Here's how the part is built. I have some questions about the finished solid (model axes, mm). A direction names the side the tool comes from. Coordinates: 2 decimals unless noted, no trailing zeros. Write each loop counter-clockwise with the first axis right and the second up, starting at its lowest first coordinate (ties: lowest second). Pieces come first, ordered by that corner, then holes. Notation, with made-up numbers: (83, 6.5) -> (107, 6.5) arc R16 ccw to (107, 10.5) -> close; hole circle Ø5 at (-24.5, -32.5). An arc over 180 degrees is marked (long way). Use a Markdown table: item, result. Add a question column.
Item 1: Imagine slicing it at C-C, the plane z = 0.3. Write out the boundary of the cut face in (x, y).
Item 2: Imagine slicing it at D-D, the plane x = 8. Write out the boundary of the cut face in (y, z).
Item 3: If we mould it in two halves opening along Y, with no side actions, what happens to faces 1 (the cylindrical face through (39.7, -10.9, 0.9)), 2 (the flat face through (36.79, 10.57, 0.89)), 3 (the flat face through (-15.78, 3, 1))? For each: pulls with the +Y half, pulls with the -Y half, needs draft (parallel to the pull), parting line crosses it, or undercut.
Item 4: Imagine slicing it at A-A, the plane x = 40. Write out the boundary of the cut face in (y, z).
Item 5: If I drill on line 1 along X through (y, z) = (-6, 0.1); line 2 along Y through (x, z) = (-9, 1.4); line 3 along Y through (x, z) = (45, 1.15) (3 decimals), over which ranges is the centre line in solid material (lowest first)? Write a range as from..to.
Item 6: Imagine slicing it at B-B, the plane y = -4. Write out the boundary of the cut face in (x, z).
Item 7: Will these pins go through, and if not, where does the flat tip stop? pin 1 Ø1 at (x, z) = (17, 0.5) entering from -Y; pin 2 Ø1 at (y, z) = (-1.5, 0) entering from +X; pin 3 Ø0.5 at (x, z) = (2.5, 1) entering from -Y.
Item 8: On a 3-axis mill with a long thin cutter (end or side, diameter ignored), from which of +Z, -Z, +X, -X, +Y, -Y can I reach the whole of each face in a straight line? I mean faces 4 (the flat face through (4, 15.405, 1)), 5 (the flat face through (-3, -9.595, 1)). Say none if no direction works.
```python
from build123d import *

# Parameters (mm, degrees)
RESSALTO_EXTRUS_O3_DEPTH = 1.8
ESBO_O7_R                = 5
CORTE_EXTRUS_O5_DEPTH    = 3


with BuildPart() as part:
    # Esboço1 → Ressalto-extrusão3 (new body)
    with BuildSketch(Plane.XY):
        with BuildLine():
            Line((-15.780332987, 15.405349819), (25.337197849, 15.405349819))
            Line((25.337197849, 15.405349819), (48.575213244, 5.595781738))
            ThreePointArc((48.575213244, 5.595781738), (51.52798537, -14.949789194), (30.790948881, -15.852377581))
            Line((30.790948881, -15.852377581), (9.828194525, -9.594650181))
            Line((9.828194525, -9.594650181), (-15.780332987, -9.594650181))
            Line((-15.780332987, -9.594650181), (-15.780332987, 15.405349819))
        make_face()
    extrude(amount=RESSALTO_EXTRUS_O3_DEPTH)

    # Esboço7 → Corte-extrusão5 (cut)
    with BuildSketch(Plane.XY.offset(1.8)):
        with Locations((40.750876667, -6.013686688)):
            Circle(ESBO_O7_R)
    extrude(amount=-CORTE_EXTRUS_O5_DEPTH, mode=Mode.SUBTRACT)


solid = part.part
```
Ans:
| question | item | result |
|---|---|---|
| 1 | outline | (-15.78, -9.59) -> (9.83, -9.59) -> (30.79, -15.85) arc R14 ccw (long way) to (48.58, 5.6) -> (25.34, 15.41) -> (-15.78, 15.41) -> close; hole circle Ø10 at (40.75, -6.01) |
| 2 | outline | (-9.59, 0) -> (15.41, 0) -> (15.41, 1.8) -> (-9.59, 1.8) -> close |
| 3 | face 1 | undercut |
| 3 | face 2 | pulls with the +Y half |
| 3 | face 3 | needs draft |
| 4 | outline | (-19.99, 0) -> (-10.96, 0) -> (-10.96, 1.8) -> (-19.99, 1.8) -> close; (-1.07, 0) -> (9.22, 0) -> (9.22, 1.8) -> (-1.07, 1.8) -> close |
| 5 | line 1 | x = -15.78..35.75, 45.75..54.75 |
| 5 | line 2 | y = -9.59..15.41 |
| 5 | line 3 | y = -19.353..-8.649, -3.378..7.105 |
| 6 | outline | (-15.78, 0) -> (36.17, 0) -> (36.17, 1.8) -> (-15.78, 1.8) -> close; (45.33, 0) -> (54.61, 0) -> (54.61, 1.8) -> (45.33, 1.8) -> close |
| 7 | pin 1 | stops at y = -11.88 |
| 7 | pin 2 | stops at x = 54.16 |
| 7 | pin 3 | stops at y = -9.59 |
| 8 | face 4 | +Z, -Z, +X, -X, +Y |
| 8 | face 5 | +Z, -Z, -X, -Y |
